Design review of the part shown in the three views and the two pictorial views. Dimensions are in mm from the part's minimum x, y and z. A direction names the side the tool comes from. Coordinates: 2 decimals unless noted, no trailing zeros. Loops run counter-clockwise (first coordinate to the right, second up) from the corner with the lowest first, then second, coordinate; pieces in that order, holes last.
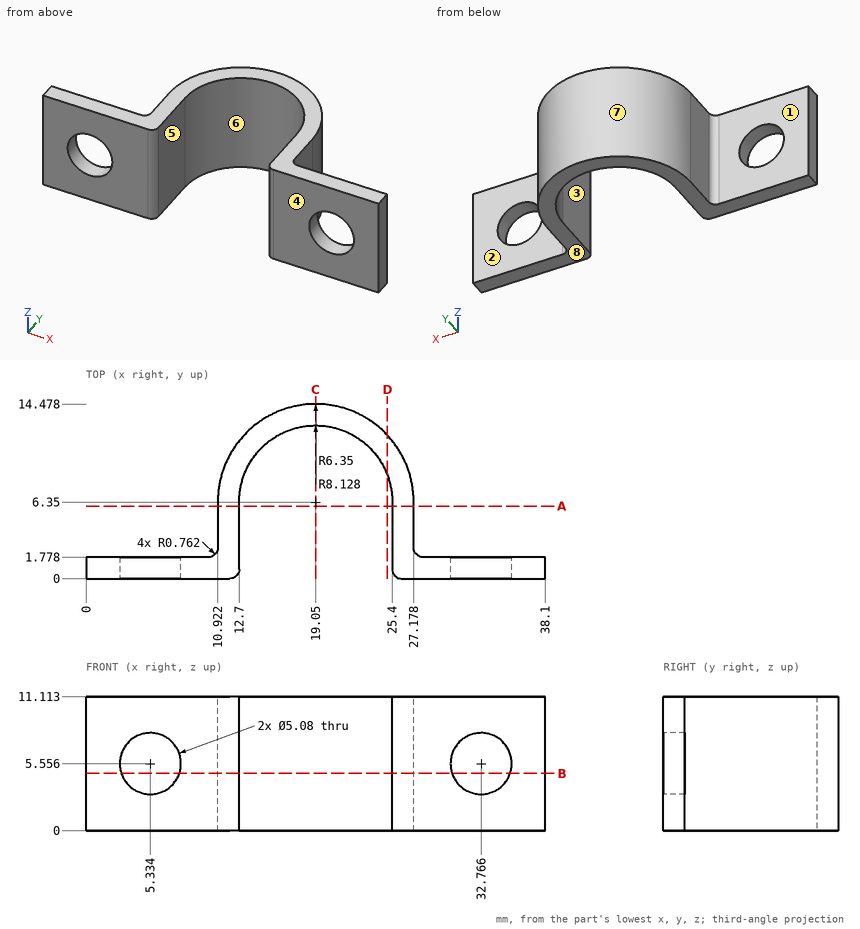
Q1. Consider section C-C (x = 19.05). State the section outline as (y, z) points.
Q2. Consider section A-A (y = 6). State the section outline as (x, z) points.
Q3. For pin 1 Ø1 at (x, z) = (34.5, 3.5) entering from +Y; pin 2 Ø4 at (y, z) = (7, 5) entering from -X; pin 3 Ø1.9 at (y, z) = (5, 5.5) entering from +X; pin 4 Ø6.5 at (x, z) = (5.33, 5.56) entering from -Y, all flat-tipped, find the tip position at first contact; note any pin that passes through.
Q4. The part is to be moulded in two halves that separate along X. For the marked faces 5, 6, 7 and 8, say which applies: +X half, -X half, draft (parallel to the pull), parting line (faces both ways), or undercut.
Q5. Machinability: for the marked faces 1, 2, 3 and 4, which of the approach directions +Z, -Z, +X, -X, +Y, -Y give a long, thin tool a straight path to every point of the face, cutting with its end or side? Answer none if there is none.
Q6. Wall thickness on probe 1 along X at (y, z) = (6.5, 8.5); probe 2 along X at (y, z) = (1, 9.5); probe 3 along Y at (x, z) = (29.5, 1.5): over which ranges is each line inside the solid? List them lowest first.
Q7. Consider section B-B (z = 4.75). Count the separate pieces of the cut face and the enclosed holes in it.
Q8. Consider section D-D (x = 25). State the section outline as (y, z) points.
Model answer:
1. outline: (12.7, 0) - (14.48, 0) - (14.48, 11.11) - (12.7, 11.11) - close
2. outline: (10.92, 0) - (12.7, 0) - (12.7, 11.11) - (10.92, 11.11) - close; (25.4, 0) - (27.18, 0) - (27.18, 11.11) - (25.4, 11.11) - close
3. pin 1: stops at y = 1.78
3. pin 2: stops at x = 10.92
3. pin 3: stops at x = 27.18
3. pin 4: stops at y = 0
4. face 5: undercut
4. face 6: undercut
4. face 7: parting line
4. face 8: draft
5. face 1: +Z, -Z, -X, +Y
5. face 2: +Z, -Z, +X, +Y
5. face 3: +Z, -Z, -Y
5. face 4: +Z, -Z, +X, -X, -Y
6. probe 1: x = 10.92 to 12.7, 25.4 to 27.18
6. probe 2: x = 0 to 12.7, 25.4 to 38.1
6. probe 3: y = 0 to 1.78
7. separate pieces: 3
7. enclosed holes: 0
8. outline: (8.57, 0) - (11.89, 0) - (11.89, 11.11) - (8.57, 11.11) - close
